```python
from build123d import *

# Parameters (mm, degrees)
IZIM1_W                     = 66.6
IZIM1_H                     = 83
Y_KSEKLIK_EKSTR_ZYON1_DEPTH = 2
Y_KSEKLIK_EKSTR_ZYON2_DEPTH = 83
Y_KSEKLIK_EKSTR_ZYON3_DEPTH = 2.3
Y_KSEKLIK_EKSTR_ZYON4_DEPTH = 2
IZIM6_R                     = 1.5
KES_EKSTR_ZYON2_DEPTH       = 4


with BuildPart() as part:
    # Çizim1 → Yükseklik-Ekstrüzyon1 (new body)
    with BuildSketch(Plane.XY):
        with Locations((33.3, 41.5)):
            Rectangle(IZIM1_W, IZIM1_H)
    extrude(amount=Y_KSEKLIK_EKSTR_ZYON1_DEPTH)

    # Çizim2 → Yükseklik-Ekstrüzyon2 (add)
    with BuildSketch(Plane(origin=(0, 83, 0), x_dir=(1, 0, 0), z_dir=(0, 1, 0))):
        with BuildLine():
            Line((0, 0), (-1, 0))
            ThreePointArc((-1, 0), (-1.707106781, -0.292893219), (-2, -1))
            Line((-2, -1), (-2, -4.85))
            ThreePointArc((-2, -4.85), (-1.414213562, -6.264213562), (0, -6.85))
            Line((0, -6.85), (1.4, -6.85))
            Line((1.4, -6.85), (1.4, -4.35))
            Line((1.4, -4.35), (0, -4.35))
            Line((0, -4.35), (0, 0))
        make_face()
        with BuildLine():
            Line((65.2, -4.35), (65.2, -6.85))
            Line((65.2, -6.85), (66.6, -6.85))
            ThreePointArc((66.6, -6.85), (68.014213562, -6.264213562), (68.6, -4.85))
            Line((68.6, -4.85), (68.6, -1))
            ThreePointArc((68.6, -1), (68.307106781, -0.292893219), (67.6, 0))
            Line((67.6, 0), (66.6, 0))
            Line((66.6, 0), (66.6, -4.35))
            Line((66.6, -4.35), (65.2, -4.35))
        make_face()
    extrude(amount=-Y_KSEKLIK_EKSTR_ZYON2_DEPTH)

    # Çizim4 → Yükseklik-Ekstrüzyon3 (add)
    with BuildSketch(Plane.XZ):
        with BuildLine():
            Line((-1, 0), (67.6, 0))
            ThreePointArc((67.6, 0), (68.307106781, 0.292893219), (68.6, 1))
            Line((68.6, 1), (68.6, 4.85))
            ThreePointArc((68.6, 4.85), (68.014213562, 6.264213562), (66.6, 6.85))
            Line((66.6, 6.85), (65.2, 6.85))
            Line((65.2, 6.85), (65.2, 4.35))
            Line((65.2, 4.35), (66.6, 4.35))
            Line((66.6, 4.35), (66.6, 2))
            Line((66.6, 2), (0, 2))
            Line((0, 2), (0, 4.35))
            Line((0, 4.35), (1.4, 4.35))
            Line((1.4, 4.35), (1.4, 6.85))
            Line((1.4, 6.85), (0, 6.85))
            ThreePointArc((0, 6.85), (-1.414213562, 6.264213562), (-2, 4.85))
            Line((-2, 4.85), (-2, 1))
            ThreePointArc((-2, 1), (-1.707106781, 0.292893219), (-1, 0))
        make_face()
    extrude(amount=Y_KSEKLIK_EKSTR_ZYON3_DEPTH)

    # Çizim5 → Yükseklik-Ekstrüzyon4 (add)
    with BuildSketch(Plane.XZ.offset(2.3)):
        with BuildLine():
            Line((67.6, 0), (-1, 0))
            ThreePointArc((-1, 0), (-1.707106781, 0.292893219), (-2, 1))
            Line((-2, 1), (-2, 8))
            Line((-2, 8), (68.6, 8))
            Line((68.6, 8), (68.6, 1))
            ThreePointArc((68.6, 1), (68.307106781, 0.292893219), (67.6, 0))
        make_face()
    extrude(amount=Y_KSEKLIK_EKSTR_ZYON4_DEPTH)

    # Çizim6 → Kes-Ekstrüzyon2 (cut)
    with BuildSketch(Plane.XZ.offset(4.3)):
        with Locations(Location((33.3, 5, 0), (0, 0, 270))):
            Circle(IZIM6_R)
    extrude(amount=-KES_EKSTR_ZYON2_DEPTH, mode=Mode.SUBTRACT)


solid = part.part
```
The model under review builds one solid part; all positions refer to its coordinate system, in mm. A direction names the side the tool comes from. Round coordinates to 2 decimals unless told otherwise and drop trailing zeros. Order: outer loops, then holes, each group sorted by start corner. A loop starts at its lowest first (then second) coordinate and runs counter-clockwise, first axis right, second up. Notation, with made-up numbers: M 33.25,83.5 L 48.25,83.5 A27 ccw 48.25,111.5 Z; hole C -8,-4 d5. An arc over 180 degrees is marked long. Use a Markdown table: item, result.
1) Tool access review of faces 1 (the face through (0, 41, 3)), 2 (the face through (-1.4, 40.95, 6.28)), 3 (the face through (1.4, 41, 6)): name each direction out of +Z, -Z, +X, -X, +Y, -Y from which nothing blocks a thin tool from reaching the whole face with its end or side.
Report:
| item | result |
|---|---|
| face 1 | +Y |
| face 2 | +Z, -X, +Y |
| face 3 | +Z, +Y |
2) Consider section C-C (x = 45.5). Write out the cut boundary in (y, z), then the cut area to 3 significant figures.
Report:
| item | result |
|---|---|
| outline | M -4.3,0 L 83,0 L 83,2 L -2.3,2 L -2.3,8 L -4.3,8 Z |
| area | 187 mm^2 |
3) Wall thickness on line 1 along X through (y, z) = (-2.85, 5); line 2 along Z through (x, y) = (25, 18); line 3 along Y through (x, z) = (42, 6.75): over which ranges is each line inside the solid? List them lowest first. Write a range as [from, to].
Report:
| item | result |
|---|---|
| line 1 | [-2, 31.8], [34.8, 68.6] |
| line 2 | [0, 2] |
| line 3 | [-4.3, -2.3] |
4) Consider section A-A (x = 33.3). Write out the cut boundary in (y, z), then the cut area to 3 significant figures.
Report:
| item | result |
|---|---|
| outline | M -4.3,0 L 83,0 L 83,2 L -2.3,2 L -2.3,3.5 L -4.3,3.5 Z; M -4.3,6.5 L -2.3,6.5 L -2.3,8 L -4.3,8 Z |
| area | 181 mm^2 |
5) Insertion check: pin 1 (3 mm diameter, centred on x = 20, y = 38.5, fed in from +Z); pin 2 (1 mm diameter, centred on x = 30, z = 7, fed in from +Y); pin 3 (1.1 mm diameter, centred on x = 66, y = 54.5, fed in from +Z). Each pin has a flat end and moves straight along its axis. Give the tip position at first contact, or say it passes through.
Report:
| item | result |
|---|---|
| pin 1 | z = 2 |
| pin 2 | y = -2.3 |
| pin 3 | z = 6.85 |
6) Consider section B-B (y = 62.5). Write out the cut boundary in (x, z), then the cut area to 3 significant figures.
Report:
| item | result |
|---|---|
| outline | M -2,1 A1 ccw -1,0 L 67.6,0 A1 ccw 68.6,1 L 68.6,4.85 A2 ccw 66.6,6.85 L 65.2,6.85 L 65.2,4.35 L 66.6,4.35 L 66.6,2 L 0,2 L 0,4.35 L 1.4,4.35 L 1.4,6.85 L 0,6.85 A2 ccw -2,4.85 Z |
| area | 165 mm^2 |
7) Draft analysis for pull direction X (two halves, no side actions). For faces 4 (the face through (33, -3, 8)), 5 (the face through (34, 41, 2)), 6 (the face through (65.2, 41, 6)), 7 (the face through (68.03, 40.95, 6.25)), state which applies: released by +X, released by -X, zero draft, split by the parting line, or undercut.
Report:
| item | result |
|---|---|
| face 4 | zero draft |
| face 5 | undercut |
| face 6 | undercut |
| face 7 | released by +X |
